Drawing for the job (mm, zero at the part's lowest x, y, z). A direction names the side the tool comes from. Round coordinates to 2 decimals unless told otherwise and drop trailing zeros. Order: outer loops, then holes, each group sorted by start corner. A loop starts at its lowest first (then second) coordinate and runs counter-clockwise, first axis right, second up. Notation, with made-up numbers: (74.5, 40) - (107.5, 40) arc R22 cw to (107.5, 49) - close; hole circle Ø10 at (67, 7.25). An arc over 180 degrees is marked (long way). Put each result on its own line as item: value. Start each with the question number.
Item 1: Mould opens along Y. For the marked faces 1, 2 and 3 say: pulls with the +Y half, pulls with the -Y half, needs draft (parallel to the pull), parting line crosses it, or undercut.
Item 2: Saw through at D-D on x = 67.5. List the corners of the cut face in (y, z).
Item 3: Pin check, flat tips, straight feed: pin 1 Ø3 at (x, z) = (61, 2) entering from -Y; pin 2 Ø1 at (y, z) = (11, 5) entering from +X; pin 3 Ø3 at (y, z) = (40, 4) entering from +X. Stop position of each tip, or through.
Item 4: Saw through at C-C on x = 47. List the corners of the cut face in (y, z).
Item 5: Probe probe 1 along X at (y, z) = (7, 3) (1 decimal); probe 2 along Y at (x, z) = (48, 3) (1 decimal); probe 3 along X at (y, z) = (25, 4.75). List the from-to ranges inside material, lowest first.
Item 6: Which spindle directions (+Z, -Z, +X, -X, +Y, -Y) get a long thin tool onto all of the face, cutting with end or side? Do the marked faces 4, 5 and 6. Say none if no direction does.
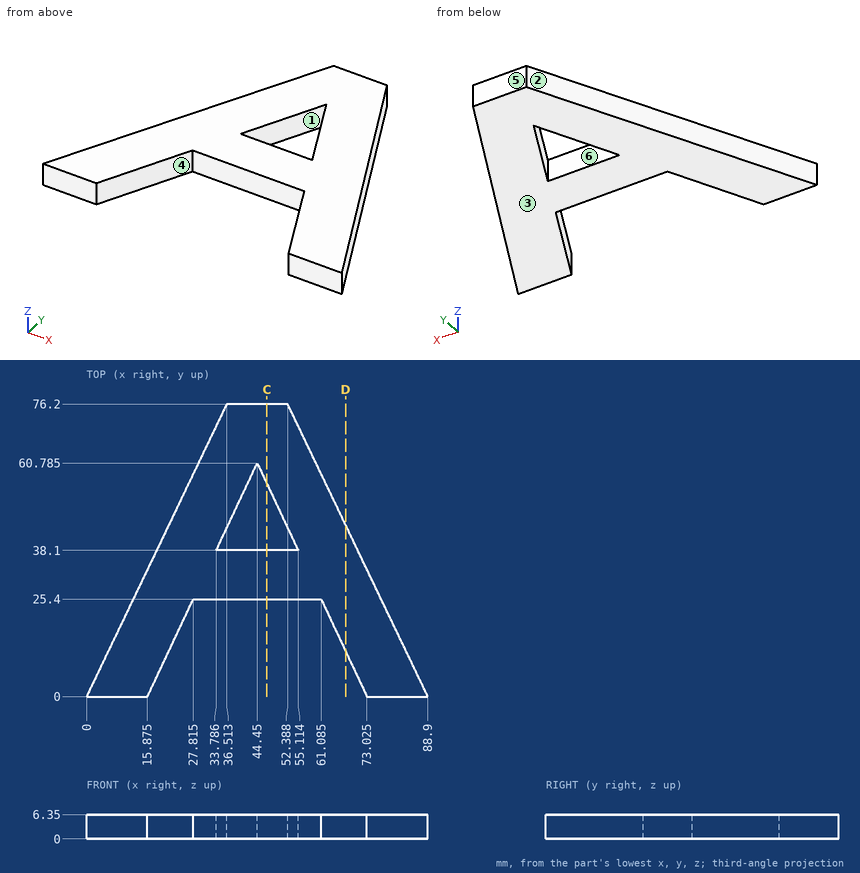
Results found:
1. face 1: undercut
1. face 2: pulls with the +Y half
1. face 3: needs draft
2. outline: (11.75, 0) - (44.66, 0) - (44.66, 6.35) - (11.75, 6.35) - close
3. pin 1: stops at y = 22.39
3. pin 2: stops at x = 83.87
3. pin 3: stops at x = 70.45
4. outline: (25.4, 0) - (38.1, 0) - (38.1, 6.35) - (25.4, 6.35) - close; (55.36, 0) - (76.2, 0) - (76.2, 6.35) - (55.36, 6.35) - close
5. probe 1: x = 3.4 to 19.2, 69.7 to 85.5
5. probe 2: y = 25.4 to 38.1, 53.2 to 76.2
5. probe 3: x = 11.98 to 27.63, 61.27 to 76.92
6. face 4: +Z, -Z, -Y
6. face 5: +Z, -Z, +X, -X, +Y
6. face 6: +Z, -Z
